Verification items for this drawing (mm, ordinates from the low corner). A direction names the side the tool comes from. Round coordinates to 2 decimals unless told otherwise and drop trailing zeros. Order: outer loops, then holes, each group sorted by start corner. A loop starts at its lowest first (then second) coordinate and runs counter-clockwise, first axis right, second up. Notation, with made-up numbers: (77.25, 50.25) - (95.25, 50.25) arc R15 cw to (95.25, 72.25) - close; hole circle Ø1 at (42, 1). An arc over 180 degrees is marked (long way). One line per question, with ' | ' between items. Start each with the question number.
Q1. Sectioned sample at C-C, the plane x = 549.5. Enter the section's corners in (y, z).
Q2. Sectioned sample at A-A, the plane z = 163.5. Enter the section's corners in (x, y), then the cut area to 3 significant figures.
Q3. Tool access check on the marked faces 1 and 2. Record the directions out of +Z, -Z, +X, -X, +Y, -Y that give a thin tool (end or side, any length) a straight path to the whole face; none if there is none.
Q4. Sectioned sample at B-B, the plane y = 102. Enter the section's corners in (x, z), then the cut area to 3 significant figures.
Q5. Material ranges on line 1 along X through (y, z) = (108, 101.5); line 2 along Z through (x, y) = (530, 25.25); line 3 along Y through (x, z) = (390, 108.5), recorded low to high.
Q6. Mould release check, pull along X, two halves, no side actions. Record for the marked faces 3, 4 and 5: +X half, -X half, draft (parallel to the pull), parting line (faces both ways), or undercut.
Q7. Gauge pin test, flat ends, axial feed: P1, Ø4.5, axis at x = 531, z = 27.5, coming from the +Y side; P2, Ø4, axis at x = 233, z = 158.5, coming from the -Y side; P3, Ø1.5, axis at x = 395, z = 88.5, coming from the +Y side. Record the tip position at first contact, or that the pin passes through.
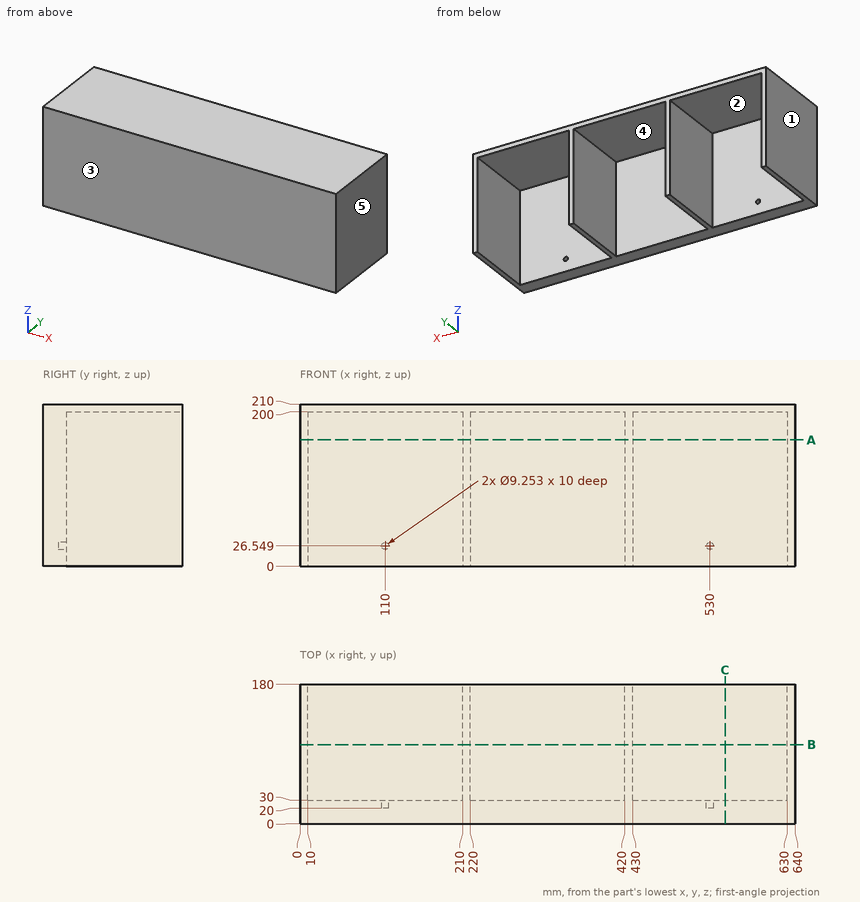
Determined:
1) outline: (0, 0) - (30, 0) - (30, 200) - (180, 200) - (180, 210) - (0, 210) - close
2) outline: (0, 0) - (640, 0) - (640, 180) - (630, 180) - (630, 30) - (430, 30) - (430, 180) - (420, 180) - (420, 30) - (220, 30) - (220, 180) - (210, 180) - (210, 30) - (10, 30) - (10, 180) - (0, 180) - close | area: 25,200 mm2
3) face 1: +Z, -Z, -X, +Y, -Y | face 2: -Z, +Y
4) outline: (0, 0) - (10, 0) - (10, 200) - (210, 200) - (210, 0) - (220, 0) - (220, 200) - (420, 200) - (420, 0) - (430, 0) - (430, 200) - (630, 200) - (630, 0) - (640, 0) - (640, 210) - (0, 210) - close | area: 14,400 mm2
5) line 1: x = 0 to 10, 210 to 220, 420 to 430, 630 to 640 | line 2: z = 0 to 21.92, 31.18 to 210 | line 3: y = 0 to 30
6) face 3: draft | face 4: undercut | face 5: +X half
7) P1: stops at y = 20 | P2: stops at y = 0 | P3: stops at y = 30
